The listing builds one solid part. Answer for the finished solid, in the listing's coordinates (mm). Coordinates: 2 decimals unless noted, no trailing zeros. Write each loop counter-clockwise with the first axis right and the second up, starting at its lowest first coordinate (ties: lowest second). Pieces come first, ordered by that corner, then holes.
from build123d import *

# Parameters (mm, degrees)
ESQUISSE1_W             = 130
ESQUISSE1_H             = 160
BOSS_EXTRU_1_DEPTH      = 1.6
ESQUISSE2_R             = 2
ENL_V_MAT_EXTRU_1_DEPTH = 104.090057717
CONG_1_R                = 5


with BuildPart() as part:
    # Esquisse1 → Boss.-Extru.1 (new body)
    with BuildSketch(Plane(origin=(0, 0, 0), x_dir=(1, 0, 0), z_dir=(0, 1, 0))):
        Rectangle(ESQUISSE1_W, ESQUISSE1_H)
    extrude(amount=BOSS_EXTRU_1_DEPTH)

    # Esquisse2 → Enlèv. mat.-Extru.1 (cut, through all)
    with BuildSketch(Plane(origin=(0, 1.6, 0), x_dir=(1, 0, 0), z_dir=(0, 1, 0))):
        with Locations(Location((-60, 73, 0), (0, 0, 270))):
            Circle(ESQUISSE2_R)
        with Locations(Location((-60, -3, 0), (0, 0, 270))):
            Circle(ESQUISSE2_R)
        with Locations(Location((-60, -73, 0), (0, 0, 270))):
            Circle(ESQUISSE2_R)
        with Locations(Location((60, -73, 0), (0, 0, 90))):
            Circle(ESQUISSE2_R)
        with Locations(Location((60, -3, 0), (0, 0, 90))):
            Circle(ESQUISSE2_R)
        with Locations(Location((60, 73, 0), (0, 0, 90))):
            Circle(ESQUISSE2_R)
    extrude(amount=-ENL_V_MAT_EXTRU_1_DEPTH, mode=Mode.SUBTRACT)

    # Congé1
    cong_1_edges = [part.edges().sort_by_distance(p)[0] for p in [
        (65, 0.8, 80),
        (-65, 0.8, 80),
        (-65, 0.8, -80),
        (65, 0.8, -80),
    ]]
    fillet(cong_1_edges, radius=CONG_1_R)


solid = part.part
1. Flat-ended cylindrical pins translate along their axes: P1, Ø3, axis at x = 60, z = 3, coming from the +Y side; P2, Ø5, axis at x = 60, z = -73, coming from the -Y side. Find the tip coordinate at first contact, or state that the pin passes through.
Results found:
P1: passes through
P2: stops at y = 0
2. For a pull along Z with two mould halves and no side action, classify faces 1 (the cylindrical face through (63, 1, -79)), 2 (the cylindrical face through (63, 1, 79)), 3 (the cylindrical face through (-58, 1, 3)) as pulls with the +Z half, pulls with the -Z half, needs draft (parallel to the pull), parting line crosses it, or undercut.
Results found:
face 1: pulls with the -Z half
face 2: pulls with the +Z half
face 3: undercut
3. Find the intervals of material crossed by L1, parallel to X at y = 0.45, z = -73; L2, parallel to Z at x = 60, y = 0.85, in increasing order.
Results found:
L1: x = -65 to -62, -58 to 58, 62 to 65
L2: z = -80 to -75, -71 to 1, 5 to 71, 75 to 80
4. Section A-A on z = 73 is taken. Give the vertices of the cut face in (x, y).
Results found:
outline: (-65, 0) - (-62, 0) - (-62, 1.6) - (-65, 1.6) - close; (-58, 0) - (58, 0) - (58, 1.6) - (-58, 1.6) - close; (62, 0) - (65, 0) - (65, 1.6) - (62, 1.6) - close
